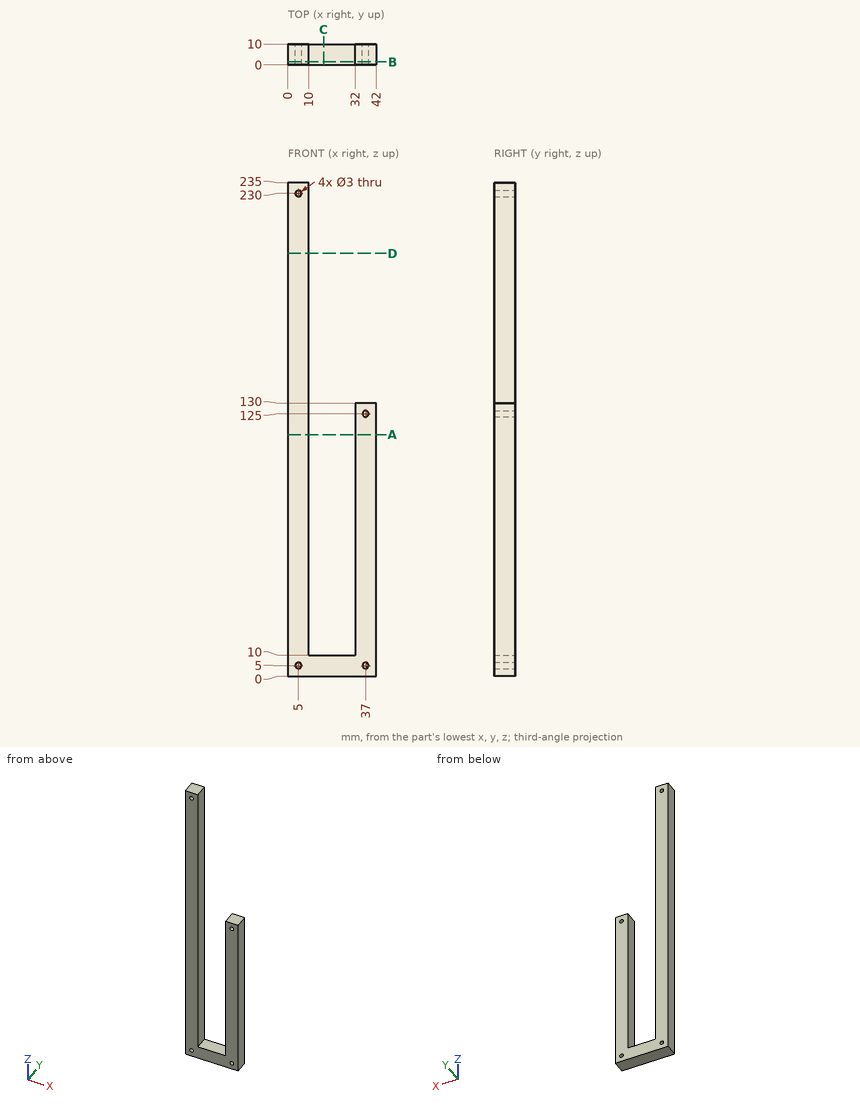
Can you work these out from the drawing? Everything is in mm from the part's minimum corner. Coordinates: 2 decimals unless noted, no trailing zeros. Loops run counter-clockwise (first coordinate to the right, second up) from the corner with the lowest first, then second, coordinate; pieces in that order, holes last. Notation, with made-up numbers: (85, 13.25) - (129, 13.25) arc R23 cw to (129, 39.25) - close; hole circle Ø9 at (45, 58). An arc over 180 degrees is marked (long way). Answer as CSV lines item,"result".
Q1. If I drill on L1, parallel to Z at x = 5, y = 5; L2, parallel to Z at x = 37, y = 2; L3, parallel to X at y = 5.5, z = 125, over which ranges is the centre line in solid material (lowest first)? Write a range as [from, to].
Response:
L1,"[0, 3.5], [6.5, 228.5], [231.5, 235]"
L2,"[0, 3.5], [6.5, 123.5], [126.5, 130]"
L3,"[0, 10], [32, 35.5], [38.5, 42]"
Q2. If we section it at C-C, the plane x = 17: Write out the boundary of the cut face in (y, z).
Response:
outline,"(0, 0) - (10, 0) - (10, 10) - (0, 10) - close"
Q3. If we section it at B-B, the plane y = 1.5: Write out the boundary of the cut face in (x, z).
Response:
outline,"(0, 0) - (42, 0) - (42, 130) - (32, 130) - (32, 10) - (10, 10) - (10, 235) - (0, 235) - close; hole circle Ø3 at (5, 5); hole circle Ø3 at (5, 230); hole circle Ø3 at (37, 5); hole circle Ø3 at (37, 125)"
Q4. If we section it at A-A, the plane z = 115: Write out the boundary of the cut face in (x, y), and give its area (3 significant figures).
Response:
outline,"(0, 0) - (10, 0) - (10, 10) - (0, 10) - close; (32, 0) - (42, 0) - (42, 10) - (32, 10) - close"
area,"200 mm2"
Q5. For pin 1 (1.5 mm diameter, centred on x = 30, y = 7.5, fed in from +Z); pin 2 (5 mm diameter, centred on x = 34.5, y = 7.5, fed in from +Z), each with a flat end and sliding along its axis, tell me the tip position at first contact or that it passes through.
Response:
pin 1,"z = 10"
pin 2,"z = 130"
